Can you work these out from the model? Positions are in its coordinate system, mm. Give positions to 0.01 mm unless a question says otherwise; leave off trailing zeros. Order: outer loops, then holes, each group sorted by start corner. A loop starts at its lowest first (then second) coordinate and runs counter-clockwise, first axis right, second up. Notation, with made-up numbers: (87, -28.5) -> (110, -28.5) arc R27 cw to (110, 5.5) -> close; hole circle Ø6 at (17, 1.5). An arc over 180 degrees is marked (long way). Answer as CSV lines item,"result".
```python
from build123d import *

# Parameters (mm, degrees)
SKETCH2_W           = 6
SKETCH2_H           = 6
BOSS_EXTRUDE1_DEPTH = 5
SKETCH3_W           = 200
SKETCH3_H           = 20
CUT_EXTRUDE1_DEPTH  = 5
SKETCH4_W           = 5
SKETCH4_H           = 5
CUT_EXTRUDE2_DEPTH  = 5


with BuildPart() as part:
    # Sketch2 → Boss-Extrude1 (new body)
    with BuildSketch(Plane.XY):
        Polygon((-100, 75), (-100, -45), (-60, -45), (-60, -65), (0, -65), (60, -65), (60, -45), (100, -45), (100, 75), align=None)
        with Locations((-55, -50)):
            Rectangle(SKETCH2_W, SKETCH2_H, mode=Mode.SUBTRACT)
        with Locations((55, -50)):
            Rectangle(SKETCH2_W, SKETCH2_H, mode=Mode.SUBTRACT)
    extrude(amount=BOSS_EXTRUDE1_DEPTH)

    # Sketch3 → Cut-Extrude1 (cut)
    with BuildSketch(Plane.XY.offset(5)):
        with Locations((0, 65)):
            Rectangle(SKETCH3_W, SKETCH3_H)
    extrude(amount=-CUT_EXTRUDE1_DEPTH, mode=Mode.SUBTRACT)

    # Sketch4 → Cut-Extrude2 (cut)
    with BuildSketch(Plane(origin=(0, 0, 0), x_dir=(-1, 0, 0), z_dir=(0, 0, -1))):
        with Locations((-97.5, 47.5)):
            Rectangle(SKETCH4_W, SKETCH4_H)
        Polygon((95, 50), (95, 45), (97.5, 45), (100, 45), (100, 50), align=None)
        with Locations((-97.5, 5)):
            Rectangle(SKETCH4_W, SKETCH4_H)
        with Locations((97.5, 5)):
            Rectangle(SKETCH4_W, SKETCH4_H)
        with Locations((-97.5, -37.5)):
            Rectangle(SKETCH4_W, SKETCH4_H)
        Polygon((100, -40), (100, -35), (95, -35), (95, -40), (97.5, -40), align=None)
    extrude(amount=-CUT_EXTRUDE2_DEPTH, mode=Mode.SUBTRACT)


solid = part.part
```
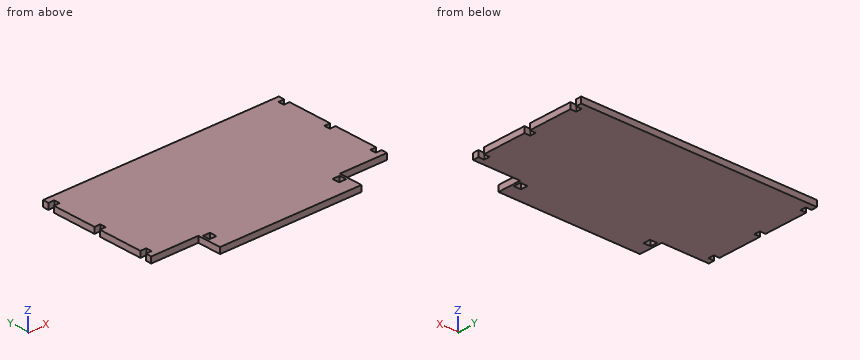
Item 1: Imagine slicing it at C-C, the plane y = 5. Please give me the cut outline in (x, z), then the cut area to 3 significant figures.
Numbers:
outline,"(-95, 0) -> (95, 0) -> (95, 5) -> (-95, 5) -> close"
area,"950 mm²"
Item 2: For pin 1 (2.5 mm diameter, centred on y = 48, z = 1.5, fed in from +X); pin 2 (2.5 mm diameter, centred on y = -50.5, z = 2, fed in from +X); pin 3 (4 mm diameter, centred on x = 47, y = 32, fed in from -Z); pin 4 (2.5 mm diameter, centred on y = -49, z = 2.5, fed in from -X), each with a flat end and sliding along its axis, tell me the tip position at first contact or that it passes through.
Numbers:
pin 1,"stops at x = 95"
pin 2,"stops at x = 60"
pin 3,"stops at z = 0"
pin 4,"stops at x = -60"
Item 3: Imagine slicing it at A-A, the plane y = -50.5. Please give me the cut outline in (x, z), then the cut area to 3 significant figures.
Numbers:
outline,"(-60, 0) -> (-58, 0) -> (-58, 5) -> (-60, 5) -> close; (-52, 0) -> (52, 0) -> (52, 5) -> (-52, 5) -> close; (58, 0) -> (60, 0) -> (60, 5) -> (58, 5) -> close"
area,"540 mm²"
Item 4: Please list where these lines run through material, in increasing order: line 1 along X through (y, z) = (-54.5, 4.8); line 2 along Y through (x, z) = (90.5, 4.75); line 3 along X through (y, z) = (5, 3.75).
Numbers:
line 1,"x = -60 to 60"
line 2,"y = -45 to 55"
line 3,"x = -95 to 95"
Item 5: Imagine slicing it at D-D, the plane x = 77.5. Please give me the cut outline in (y, z).
Numbers:
outline,"(-45, 0) -> (55, 0) -> (55, 5) -> (-45, 5) -> close"
Item 6: Imagine slicing it at B-B, the plane z = 2.35. Give the number of separate pieces and of enclosed holes in the cut face, then the cut area to 3 significant figures.
Numbers:
separate pieces,"1"
enclosed holes,"2"
area,"22,200 mm²"
